Input: part model. Units: mm. Frame: model coordinates. Round coordinates to 2 decimals unless told otherwise and drop trailing zeros. Loops run counter-clockwise (first coordinate to the right, second up) from the corner with the lowest first, then second, coordinate; pieces in that order, holes last. Notation, with made-up numbers: (78, -25) - (91, -25) arc R7 cw to (91, -19) - close; hole circle Ø3 at (-30.5, 10). An arc over 180 degrees is marked (long way). One line per question, with ' | ' between items. Start each with the question number.
Item 1: Section B-B, the plane y = -32.5. Return loops of the section in (x, z), plus the area to 3 significant figures.
Item 2: First-contact query: pin 1 (4 mm diameter, centred on x = -135, y = -240, fed in from +Z); pin 2 (1 mm diameter, centred on y = 13, z = 0.5, fed in from -X). Flat tips, straight axial feed; report the tip coordinate or a pass-through.
Item 3: Section A-A, the plane x = 50.5. Return loops of the section in (y, z), plus the area to 3 significant figures.
Item 4: Material intervals for line 1 along X through (y, z) = (5.5, 1.4); line 2 along X through (y, z) = (5, 0.75); line 3 along Y through (x, z) = (-135, 1.1), sorted ascending.
Item 5: Section C-C, the plane z = 1.65. Return loops of the section in (x, y), plus the area to 3 significant figures.
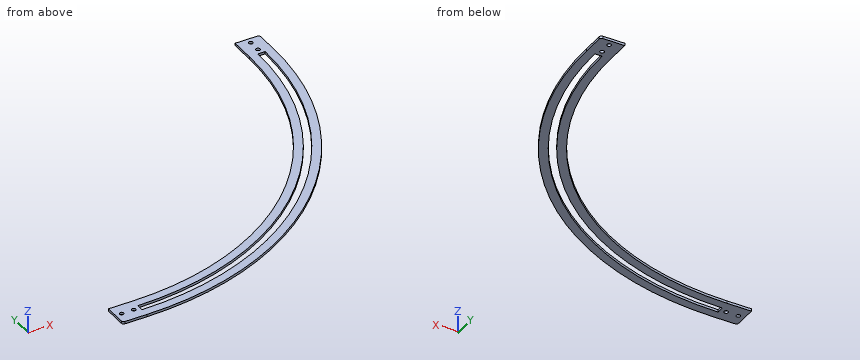
Autodesk Inventor part; units mm, degrees
ref_plane "YZ Plane" through (0, 0, 0) normal (1, 0, 0) x (0, 1, 0)
ref_plane "XZ Plane" through (0, 0, 0) normal (0, 1, 0) x (-1, 0, 0)
ref_plane "XY Plane" through (0, 0, 0) normal (0, 0, 1) x (1, 0, 0)
sketch "スケッチ1" plane through (0, 0, 0) normal (0, 0, 1) x (1, 0, 0)
  line L0 (120, -35) -> (-120, -35)
  line L1 (-120, -35) -> (-120, 35)
  line L2 (-120, 35) -> (120, 35)
  line L3 (120, 35) -> (120, -35)
  line L4 (120, -35) -> (-120, 35) construction
  line L5 (-120, -35) -> (120, 35) construction
  line L6 (-110, -35) -> (-130, -35)
  line L7 (-130, -35) -> (-130, 75)
  line L8 (-130, 75) -> (-110, 75)
  line L9 (-110, 75) -> (-110, -35)
  line L10 (110, 35) -> (130, 35)
  circle A0 centre (-120, 0) radius 6
  line L11 (110, 35) -> (130, 35)
  arc A1 (-120, -240) -> (120, 0) centre (-120, 0) ccw
  arc A2 (-120, -250) -> (130, 0) centre (-120, 0) ccw
  arc A3 (-120, -230) -> (110, 0) centre (-120, 0) ccw
  line L12 (110, 0) -> (130, 0)
  line L13 (130, 0) -> (130, 20)
  line L14 (130, 20) -> (110, 20)
  line L15 (110, 20) -> (110, 0)
  line L16 (-120, -250) -> (-140, -250)
  line L17 (-140, -250) -> (-140, -230)
  line L18 (-140, -230) -> (-120, -230)
  line L19 (-120, -230) -> (-120, -250)
  arc A4 (-120, -243) -> (123, 0) centre (-120, 0) ccw
  arc A5 (-120, -237) -> (117, 0) centre (-120, 0) ccw
  line L20 (130, 20) -> (-140, 20)
  line L21 (-140, 20) -> (-140, -250)
  line L22 (-140, -250) -> (130, -250)
  line L23 (130, -250) -> (130, 20)
  line L24 (-120, -250) -> (-120, 0)
  line L25 (-120, 0) -> (130, 0)
  point P0 (0, 0)
  point P1 (120, 25)
  point P2 (117, 0)
  point P3 (123, 0)
  point P4 (-120, -243)
  point P5 (-120, -237)
  dimension "d0" = 240
  dimension "d1" = 70
  dimension "d2" = 20
  dimension "d3" = 110
  dimension "d4" = 10
  dimension "d8" = 12
  dimension "d14" = 10
  dimension "d18" = 10
  dimension "d19" = 10
  dimension "d20" = 20
  dimension "d21" = 20
  dimension "d22" = 20
  dimension "d23" = 20
  dimension "d26" = 3
  dimension "d27" = 3
  dimension "d37" = 20
extrude "押し出し1" add sketch "スケッチ1" along normal blind 2 contours A3 L12 A5 L0 | L0 A5 L19 A3 | L19 L16 L17 L18 | L15 L14 L3 L12 | L3 L14 L13 L12 | L19 A4 L12 A2
sketch "スケッチ2" plane through (0, 0, 2) normal (0, 0, 1) x (1, 0, 0)
  line L0 (130, 20) -> (110, 20)
  line L1 (120, 20) -> (120, 0)
  line L2 (117, 0) -> (123, 0)
  line L3 (-140, -230) -> (-140, -250)
  line L4 (-140, -240) -> (-120, -240)
  point P0 (0, 0)
  point P1 (120, 15)
  point P2 (120, 5)
  point P3 (-135, -240)
  point P4 (-125, -240)
  dimension "d28" = 10
  dimension "d29" = 5
  dimension "d52" = 10
  dimension "d53" = 5
hole "穴1" at (120, 15, 2) at (120, 5, 2) at (-125, -240, 2) at (-135, -240, 2) direction (0, 0, -1) diameter 3.4 end through all
fillet "フィレット1" radius 2 2 edges at (130, 20, 1) (-140, -250, 1)
sketch "スケッチ5" plane through (0, 0, 2) normal (0, 0, 1) x (1, 0, 0)
  arc A0 (-140, -248) -> (-138, -250) centre (-138, -248) ccw
  line L0 (-138, -250) -> (-120, -250)
  arc A1 (-120, -250) -> (130, 0) centre (-120, 0) ccw
  line L1 (130, 0) -> (130, 18)
  arc A2 (130, 18) -> (128, 20) centre (128, 18) ccw
  line L2 (128, 20) -> (110, 20)
  line L3 (110, 20) -> (110, 0)
  arc A3 (-120, -230) -> (110, 0) centre (-120, 0) ccw
  line L4 (-120, -230) -> (-140, -230)
  line L5 (-140, -230) -> (-140, -248)
  circle A4 centre (-135, -240) radius 1.7
  circle A5 centre (-125, -240) radius 1.7
  circle A6 centre (120, 5) radius 1.7
  circle A7 centre (120, 15) radius 1.7
  line L6 (117, 0) -> (123, 0)
  arc A8 (-120, -243) -> (123, 0) centre (-120, 0) ccw
  line L7 (-120, -243) -> (-120, -237)
  arc A9 (-120, -237) -> (117, 0) centre (-120, 0) ccw
  point P0 (0, 0)
equation "\"d4\" = 0.5 * d2"
equation "\"d27\" = d26"
properties part number "xx_memo"
Return value:
1) outline: (107.69, 0) - (114.76, 0) - (114.76, 2) - (107.69, 2) - close; (120.82, 0) - (127.88, 0) - (127.88, 2) - (120.82, 2) - close | area: 28.3 mm2
2) pin 1: z = 2 | pin 2: x = 110
3) outline: (-182.84, 0) - (-173.14, 0) - (-173.14, 2) - (-182.84, 2) - close; (-164.62, 0) - (-154.37, 0) - (-154.37, 2) - (-164.62, 2) - close | area: 39.9 mm2
4) line 1: 110 to 118.38, 121.62 to 130 | line 2: 110 to 118.3, 121.7 to 130 | line 3: -250 to -241.7, -238.3 to -230
5) outline: (-140, -248) arc R2 ccw to (-138, -250) - (-120, -250) arc R250 ccw to (130, 0) - (130, 18) arc R2 ccw to (128, 20) - (110, 20) - (110, 0) arc R230 cw to (-120, -230) - (-140, -230) - close; hole circle Ø3.4 at (-135, -240); hole circle Ø3.4 at (-125, -240); hole (-120, -243) arc R243 ccw to (123, 0) - (117, 0) arc R237 cw to (-120, -237) - close; hole circle Ø3.4 at (120, 5); hole circle Ø3.4 at (120, 15) | area: 6,040 mm2
